Geometry check sheet. Reference: the model listing, model coordinates, mm. Face numbers are marked on the shaded views. A direction names the side the tool comes from. Give positions to 0.01 mm unless a question says otherwise; leave off trailing zeros. Order: outer loops, then holes, each group sorted by start corner. A loop starts at its lowest first (then second) coordinate and runs counter-clockwise, first axis right, second up.
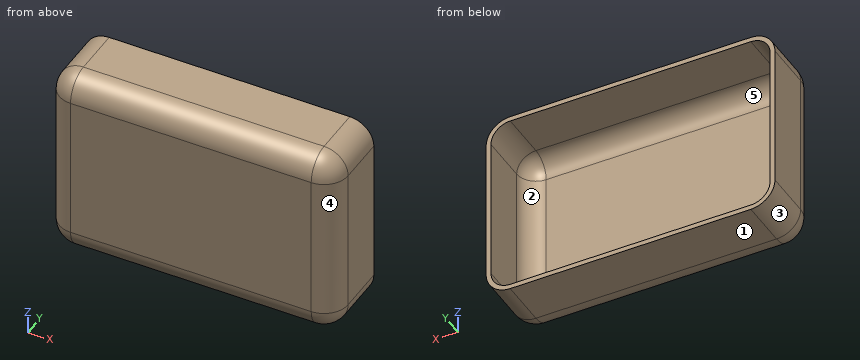
```python
from build123d import *

# Parameters (mm, degrees)
CROQUIS1_W              = 152.4
CROQUIS1_H              = 101.6
SALIENTE_EXTRUIR1_DEPTH = 38.1
REDONDEO1_R             = 12.7
VACIADO1_T              = -2.54


with BuildPart() as part:
    # Croquis1 → Saliente-Extruir1 (new body)
    with BuildSketch(Plane(origin=(0, 0, 0), x_dir=(1, 0, 0), z_dir=(0, 1, 0))):
        Rectangle(CROQUIS1_W, CROQUIS1_H)
    extrude(amount=SALIENTE_EXTRUIR1_DEPTH)

    # Redondeo1
    redondeo1_edges = [part.edges().sort_by_distance(p)[0] for p in [
        (0, 0, -50.8),
        (76.2, 0, 0),
        (0, 0, 50.8),
        (-76.2, 0, 0),
        (-76.2, 19.05, -50.8),
        (76.2, 19.05, -50.8),
        (76.2, 19.05, 50.8),
        (-76.2, 19.05, 50.8),
    ]]
    fillet(redondeo1_edges, radius=REDONDEO1_R)

    # Vaciado1
    vaciado1_openings = [part.faces().sort_by_distance(p)[0] for p in [
        (0, 38.1, 0),
    ]]
    offset(amount=VACIADO1_T, openings=vaciado1_openings, kind=Kind.INTERSECTION)


solid = part.part
```
Q1. Cross-section at D-D, the plane y = 10. Record the boundary of the cut face in (x, z), and give its area (3 significant figures).
Q2. Thickness scan on L1, parallel to Z at x = 46.5, y = 17; L2, parallel to X at y = 35, z = 11; L3, parallel to Y at x = 63, z = 18. Record the ranges inside material, lowest first.
Q3. Release check for a two-part mould opening along Z. For the marked faces 3, 4 and 5 record: pulls with the +Z half, pulls with the -Z half, needs draft (parallel to the pull), parting line crosses it, or undercut.
Q4. Cross-section at B-B, the plane z = 30. Record the boundary of the cut face in (x, y), and give its area (3 significant figures).
Q5. Cross-section at C-C, the plane x = -48. Record the boundary of the cut face in (y, z), and give its area (3 significant figures).
Q6. Access from +Z, -Z, +X, -X, +Y, -Y to the whole of each face (thin tool, end or side, straight path). Record for the marked faces 1 and 2.
Q7. Cross-section at A-A, the plane y = 35. Record the boundary of the cut face in (x, z), and give its area (3 significant figures).
Answers follow:
1. outline: (-75.91, -38.1) arc R12.41 ccw to (-63.5, -50.51) - (63.5, -50.51) arc R12.41 ccw to (75.91, -38.1) - (75.91, 38.1) arc R12.41 ccw to (63.5, 50.51) - (-63.5, 50.51) arc R12.41 ccw to (-75.91, 38.1) - close; hole (-73.29, -38.1) arc R9.79 ccw to (-63.5, -47.89) - (63.5, -47.89) arc R9.79 ccw to (73.29, -38.1) - (73.29, 38.1) arc R9.79 ccw to (63.5, 47.89) - (-63.5, 47.89) arc R9.79 ccw to (-73.29, 38.1) - close
1. area: 1,250 mm2
2. L1: z = -50.8 to -48.26, 48.26 to 50.8
2. L2: x = -76.2 to -73.66, 73.66 to 76.2
2. L3: y = 0 to 2.54
3. face 3: pulls with the -Z half
3. face 4: needs draft
3. face 5: undercut
4. outline: (-76.2, 12.7) arc R12.7 ccw to (-63.5, 0) - (63.5, 0) arc R12.7 ccw to (76.2, 12.7) - (76.2, 38.1) - (73.66, 38.1) - (73.66, 12.7) arc R10.16 cw to (63.5, 2.54) - (-63.5, 2.54) arc R10.16 cw to (-73.66, 12.7) - (-73.66, 38.1) - (-76.2, 38.1) - close
4. area: 543 mm2
5. outline: (0, -38.1) arc R12.7 ccw to (12.7, -50.8) - (38.1, -50.8) - (38.1, -48.26) - (12.7, -48.26) arc R10.16 cw to (2.54, -38.1) - (2.54, 38.1) arc R10.16 cw to (12.7, 48.26) - (38.1, 48.26) - (38.1, 50.8) - (12.7, 50.8) arc R12.7 ccw to (0, 38.1) - close
5. area: 414 mm2
6. face 1: -Z, +X, -X, +Y, -Y
6. face 2: +Y
7. outline: (-76.2, -38.1) arc R12.7 ccw to (-63.5, -50.8) - (63.5, -50.8) arc R12.7 ccw to (76.2, -38.1) - (76.2, 38.1) arc R12.7 ccw to (63.5, 50.8) - (-63.5, 50.8) arc R12.7 ccw to (-76.2, 38.1) - close; hole (-73.66, -38.1) arc R10.16 ccw to (-63.5, -48.26) - (63.5, -48.26) arc R10.16 ccw to (73.66, -38.1) - (73.66, 38.1) arc R10.16 ccw to (63.5, 48.26) - (-63.5, 48.26) arc R10.16 ccw to (-73.66, 38.1) - close
7. area: 1,210 mm2
